Check sheet for the drawn part. Datum: minimum x, y, z corner. Units: mm. A direction names the side the tool comes from. Round coordinates to 2 decimals unless told otherwise and drop trailing zeros. Write each loop counter-clockwise with the first axis right and the second up, starting at its lowest first coordinate (ties: lowest second). Pieces come first, ordered by that corner, then holes. Notation, with made-up numbers: (8, 44) - (12, 44) arc R29 ccw to (12, 67) - close; hole circle Ø3 at (25, 74). An arc over 180 degrees is marked (long way). Answer as a JSON object with one key per item and string values.
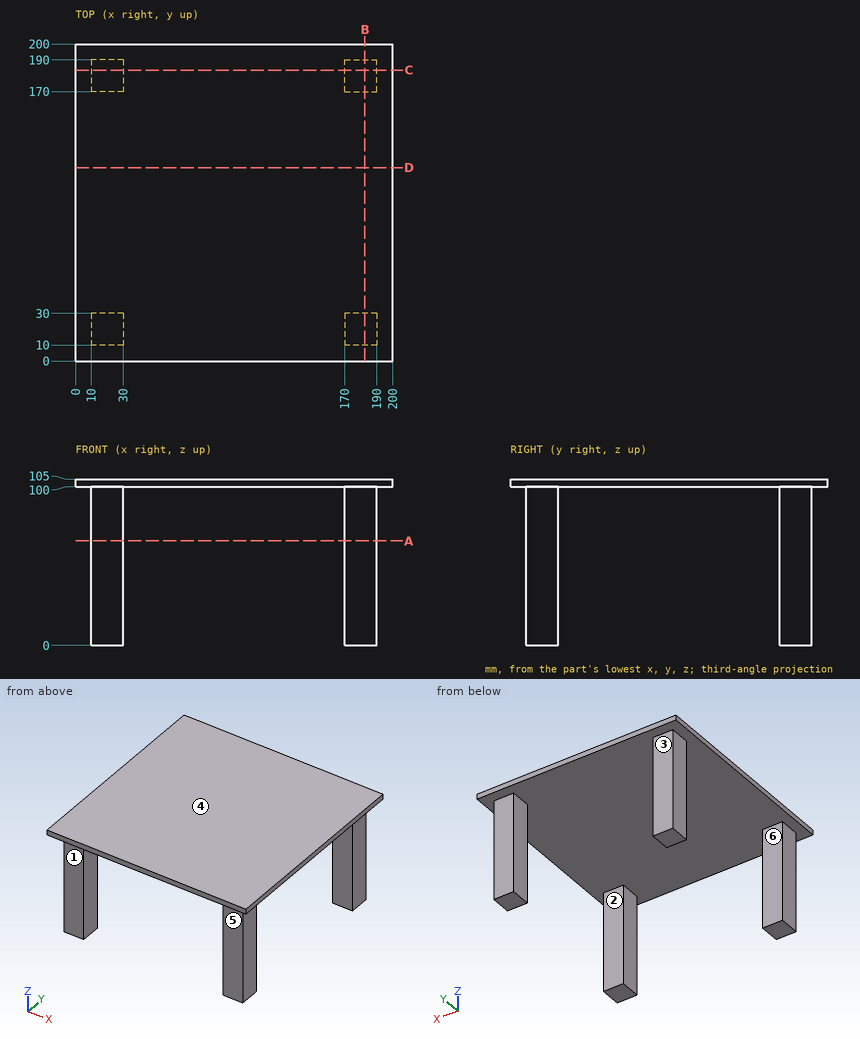
1. Cross-section at A-A (z = 66). Record the boundary of the cut face in (x, y), plus the area to 3 significant figures.
Completed:
{"outline": "(10, 10) - (30, 10) - (30, 30) - (10, 30) - close; (10, 170) - (30, 170) - (30, 190) - (10, 190) - close; (170, 10) - (190, 10) - (190, 30) - (170, 30) - close; (170, 170) - (190, 170) - (190, 190) - (170, 190) - close", "area": "1,600 mm^2"}
2. Access from +Z, -Z, +X, -X, +Y, -Y to the whole of each face (thin tool, end or side, straight path). Record for the marked faces 1, 2 and 3.
Completed:
{"face 1": "-Z, +X, -X, -Y", "face 2": "-Z, +X, -X", "face 3": "-Z, +X, -X, +Y"}
3. Mould release check, pull along Y, two halves, no side actions. Record for the marked faces 4, 5 and 6: released by +Y, released by -Y, zero draft, split by the parting line, or undercut.
Completed:
{"face 4": "zero draft", "face 5": "released by -Y", "face 6": "undercut"}
4. Material ranges on probe 1 along X at (y, z) = (184.5, 43); probe 2 along Z at (x, y) = (86, 144.5), recorded low to high. Write a range as from..to.
Completed:
{"probe 1": "x = 10..30, 170..190", "probe 2": "z = 100..105"}
5. Go/stop test with flat-tipped pins: pin 1 (5 mm diameter, centred on x = 22, y = 136, fed in from -Z); pin 2 (6 mm diameter, centred on x = 180.5, z = 28.5, fed in from +Y); pin 3 (22 mm diameter, centred on x = 183.5, z = 38, fed in from -Y). Record where each tip stops, or that it passes through.
Completed:
{"pin 1": "stops at z = 100", "pin 2": "stops at y = 190", "pin 3": "stops at y = 10"}
6. Cross-section at B-B (x = 182.5). Record the boundary of the cut face in (y, z).
Completed:
{"outline": "(0, 100) - (10, 100) - (10, 0) - (30, 0) - (30, 100) - (170, 100) - (170, 0) - (190, 0) - (190, 100) - (200, 100) - (200, 105) - (0, 105) - close"}
7. Cross-section at D-D (y = 122). Record the boundary of the cut face in (x, z), plus the area to 3 significant figures.
Completed:
{"outline": "(0, 100) - (200, 100) - (200, 105) - (0, 105) - close", "area": "1,000 mm^2"}
